Model file for the job. Use its own axes, mm. A direction names the side the tool comes from. Round coordinates to 2 decimals unless told otherwise and drop trailing zeros. Order: outer loops, then holes, each group sorted by start corner. A loop starts at its lowest first (then second) coordinate and runs counter-clockwise, first axis right, second up. Notation, with made-up numbers: (25.25, 49) -> (47.25, 49) arc R24 ccw to (47.25, 61) -> close; hole circle Ø6 at (14.5, -35). An arc over 180 degrees is marked (long way). Use CSV: the item, a comma, the result in double quotes.
```python
from build123d import *

# Parameters (mm, degrees)
SKIZZE2_W                        = 120
SKIZZE2_H                        = 39.364160046
AUFSATZ_LINEAR_AUSTRAGEN1_DEPTH  = 30
SKIZZE24_R                       = 1.55
SCHNITT_LINEAR_AUSTRAGEN4_DEPTH  = 130.805766806
SKIZZE46_R                       = 2.85
SCHNITT_LINEAR_AUSTRAGEN15_DEPTH = 10
SCHNITT_LINEAR_START             = -5
SCHNITT_LINEAR_AUSTRAGEN25_DEPTH = 2.7
LINEARES_MUSTER1_COUNT           = 4
LINEARES_MUSTER1_PITCH           = 20
SPIEGELN2_COPY_1_SKETCH_R        = 2.85
SPIEGELN2_COPY_1_DEPTH           = 10
SPIEGELN2_COPY_2_SKETCH_R        = 2.85
SPIEGELN2_COPY_2_DEPTH           = 10
SPIEGELN2_COPY_3_SKETCH_R        = 2.85
SPIEGELN2_COPY_3_DEPTH           = 10
SPIEGELN2_START                  = -5
SPIEGELN2_COPY_4_DEPTH           = 2.7
SPIEGELN2_COPY_5_DEPTH           = 2.7
SPIEGELN2_COPY_6_DEPTH           = 2.7
SKIZZE51_R                       = 1.55
SCHNITT_LINEAR_AUSTRAGEN26_DEPTH = 130.805766806
SKIZZE75_R                       = 0.75
SCHNITT_LINEAR_AUSTRAGEN28_DEPTH = 10
SKIZZE76_R                       = 2
SCHNITT_LINEAR_AUSTRAGEN29_DEPTH = 6
SKIZZE80_R                       = 0.5
SCHNITT_LINEAR_AUSTRAGEN34_DEPTH = 21
SCHNITT_LINEAR_START_2           = -7.5
SKIZZE81_R                       = 0.5
SCHNITT_LINEAR_AUSTRAGEN36_DEPTH = 5
ABSPALTEN3_OUTLINE_W             = 120
ABSPALTEN3_OUTLINE_H             = 39.364160046
ABSPALTEN3_OUTLINE_R             = 1.55
ABSPALTEN3_DEPTH                 = 15


# Read off the part's stored shape, not the designer's step: Abspalten3
with BuildPart() as part:
    # Skizze2 → Aufsatz-Linear austragen1 (new body)
    with BuildSketch(Plane.XY):
        with Locations((60, 19.682080023)):
            Rectangle(SKIZZE2_W, SKIZZE2_H)
    extrude(amount=AUFSATZ_LINEAR_AUSTRAGEN1_DEPTH)

    # Skizze24 → Schnitt-Linear austragen4 (cut, through all)
    with BuildSketch(Plane.XY.offset(30)):
        with Locations((40, 31.364160046)):
            Circle(SKIZZE24_R)
        with Locations((60, 31.364160046)):
            Circle(SKIZZE24_R)
        with Locations((80, 31.364160046)):
            Circle(SKIZZE24_R)
        with Locations((100, 31.364160046)):
            Circle(SKIZZE24_R)
    schnitt_linear_austragen4 = extrude(amount=-SCHNITT_LINEAR_AUSTRAGEN4_DEPTH, mode=Mode.SUBTRACT)

    # Skizze46 → Schnitt-Linear austragen15 (cut)
    with BuildSketch(Plane(origin=(0, 0, 0), x_dir=(-1, 0, 0), z_dir=(0, 0, -1))):
        with Locations((-100, 31.364160046)):
            Circle(SKIZZE46_R)
    schnitt_linear_austragen15 = extrude(amount=-SCHNITT_LINEAR_AUSTRAGEN15_DEPTH, mode=Mode.SUBTRACT)

    # Skizze50 → Schnitt-Linear austragen25 (cut)
    with BuildSketch(Plane.XY.offset(30).offset(SCHNITT_LINEAR_START)):
        Polygon((97.15, 33.009608314), (97.15, 39.364160046), (102.85, 39.364160046), (102.85, 33.009608314), (102.85, 29.718711779), (100, 28.073263512), (97.15, 29.718711779), align=None)
    schnitt_linear_austragen25 = extrude(amount=-SCHNITT_LINEAR_AUSTRAGEN25_DEPTH, mode=Mode.SUBTRACT)

    # Lineares Muster1: Schnitt-Linear austragen15, Schnitt-Linear austragen25 ×4
    with Locations(*[(-i * LINEARES_MUSTER1_PITCH, 0, 0) for i in range(1, LINEARES_MUSTER1_COUNT)]):
        add(schnitt_linear_austragen15, mode=Mode.SUBTRACT)
        add(schnitt_linear_austragen25, mode=Mode.SUBTRACT)

    # Spiegeln2: Schnitt-Linear austragen15, Schnitt-Linear austragen25 across plane
    add(schnitt_linear_austragen15.mirror(Plane.ZX.offset(19.764160046)), mode=Mode.SUBTRACT)
    add(schnitt_linear_austragen25.mirror(Plane.ZX.offset(19.764160046)), mode=Mode.SUBTRACT)

    # Spiegeln2 copy 1 sketch → Spiegeln2 copy 1 (cut)
    with BuildSketch(Plane(origin=(-20, 39.528320093, 0), x_dir=(-1, 0, 0), z_dir=(0, 0, -1))):
        with Locations((-100, -31.364160046)):
            Circle(SPIEGELN2_COPY_1_SKETCH_R)
    extrude(amount=-SPIEGELN2_COPY_1_DEPTH, mode=Mode.SUBTRACT)

    # Spiegeln2 copy 2 sketch → Spiegeln2 copy 2 (cut)
    with BuildSketch(Plane(origin=(-40, 39.528320093, 0), x_dir=(-1, 0, 0), z_dir=(0, 0, -1))):
        with Locations((-100, -31.364160046)):
            Circle(SPIEGELN2_COPY_2_SKETCH_R)
    extrude(amount=-SPIEGELN2_COPY_2_DEPTH, mode=Mode.SUBTRACT)

    # Spiegeln2 copy 3 sketch → Spiegeln2 copy 3 (cut)
    with BuildSketch(Plane(origin=(-60, 39.528320093, 0), x_dir=(-1, 0, 0), z_dir=(0, 0, -1))):
        with Locations((-100, -31.364160046)):
            Circle(SPIEGELN2_COPY_3_SKETCH_R)
    extrude(amount=-SPIEGELN2_COPY_3_DEPTH, mode=Mode.SUBTRACT)

    # Spiegeln2 copy 4 sketch → Spiegeln2 copy 4 (cut)
    with BuildSketch(Plane(origin=(-20, 39.528320093, 30), x_dir=(1, 0, 0), z_dir=(0, 0, 1)).offset(SPIEGELN2_START)):
        Polygon((97.15, -33.009608314), (97.15, -39.364160046), (102.85, -39.364160046), (102.85, -33.009608314), (102.85, -29.718711779), (100, -28.073263512), (97.15, -29.718711779), align=None)
    extrude(amount=-SPIEGELN2_COPY_4_DEPTH, mode=Mode.SUBTRACT)

    # Spiegeln2 copy 5 sketch → Spiegeln2 copy 5 (cut)
    with BuildSketch(Plane(origin=(-40, 39.528320093, 30), x_dir=(1, 0, 0), z_dir=(0, 0, 1)).offset(SPIEGELN2_START)):
        Polygon((97.15, -33.009608314), (97.15, -39.364160046), (102.85, -39.364160046), (102.85, -33.009608314), (102.85, -29.718711779), (100, -28.073263512), (97.15, -29.718711779), align=None)
    extrude(amount=-SPIEGELN2_COPY_5_DEPTH, mode=Mode.SUBTRACT)

    # Spiegeln2 copy 6 sketch → Spiegeln2 copy 6 (cut)
    with BuildSketch(Plane(origin=(-60, 39.528320093, 30), x_dir=(1, 0, 0), z_dir=(0, 0, 1)).offset(SPIEGELN2_START)):
        Polygon((97.15, -33.009608314), (97.15, -39.364160046), (102.85, -39.364160046), (102.85, -33.009608314), (102.85, -29.718711779), (100, -28.073263512), (97.15, -29.718711779), align=None)
    extrude(amount=-SPIEGELN2_COPY_6_DEPTH, mode=Mode.SUBTRACT)

    # Spiegeln3: Schnitt-Linear austragen4 across plane
    add(schnitt_linear_austragen4.mirror(Plane.ZX.offset(19.764160046)), mode=Mode.SUBTRACT)

    # Skizze51 → Schnitt-Linear austragen26 (cut, through all)
    with BuildSketch(Plane.XY.offset(30)):
        with Locations((5, 34.364160046)):
            Circle(SKIZZE51_R)
        with Locations((115, 5)):
            Circle(SKIZZE51_R)
    extrude(amount=-SCHNITT_LINEAR_AUSTRAGEN26_DEPTH, mode=Mode.SUBTRACT)

    # Skizze73 → Schnitt-Rotation5 (revolve, cut)
    with BuildSketch(Plane.XY.offset(15)):
        Polygon((15, 19.764160046), (15, 23.764160046), (20, 23.764160046), (20, 24.764160046), (100, 23.182080023), (100, 22.182080023), (105, 22.182080023), (105, 19.682080023), align=None)
    revolve(axis=Axis((105, 19.682080023, 15), (-0.9999995841280241, 0.0009119998787298228, 0)), mode=Mode.SUBTRACT)

    # Skizze75 → Schnitt-Linear austragen28 (cut)
    with BuildSketch(Plane.XY.offset(30)):
        with Locations((21.598259807, 19.682080023)):
            Circle(SKIZZE75_R)
    extrude(amount=-SCHNITT_LINEAR_AUSTRAGEN28_DEPTH, mode=Mode.SUBTRACT)

    # Skizze76 → Schnitt-Linear austragen29 (cut)
    with BuildSketch(Plane.XY.offset(30)):
        with Locations((21.598259807, 19.682080023)):
            Circle(SKIZZE76_R)
    extrude(amount=-SCHNITT_LINEAR_AUSTRAGEN29_DEPTH, mode=Mode.SUBTRACT)

    # Skizze80 → Schnitt-Linear austragen34 (cut)
    with BuildSketch(Plane(origin=(120, 0, 0), x_dir=(0, 0, -1), z_dir=(1, 0, 0))):
        with Locations((-22.000416524, 19.763714623)):
            Circle(SKIZZE80_R)
    schnitt_linear_austragen34 = extrude(amount=-SCHNITT_LINEAR_AUSTRAGEN34_DEPTH, mode=Mode.SUBTRACT)

    # Skizze81 → Schnitt-Linear austragen36 (cut)
    with BuildSketch(Plane.XY.offset(30).offset(SCHNITT_LINEAR_START_2)):
        with Locations(Location((99, 19.682080023, 0), (0, 0, 7.034090001))):
            Circle(SKIZZE81_R)
    schnitt_linear_austragen36 = extrude(amount=-SCHNITT_LINEAR_AUSTRAGEN36_DEPTH, mode=Mode.SUBTRACT)

    # Spiegeln4: Schnitt-Linear austragen34, Schnitt-Linear austragen36 across plane
    add(schnitt_linear_austragen34.mirror(Plane.XY.offset(15)), mode=Mode.SUBTRACT)
    add(schnitt_linear_austragen36.mirror(Plane.XY.offset(15)), mode=Mode.SUBTRACT)

    # Abspalten3 outline → Abspalten3 (cut)
    with BuildSketch(Plane.XY):
        with Locations((60, 19.682080023)):
            Rectangle(ABSPALTEN3_OUTLINE_W, ABSPALTEN3_OUTLINE_H)
        with Locations((115, 5)):
            Circle(ABSPALTEN3_OUTLINE_R, mode=Mode.SUBTRACT)
        with Locations((5, 34.364160046)):
            Circle(ABSPALTEN3_OUTLINE_R, mode=Mode.SUBTRACT)
        with Locations((40, 8.164160046)):
            Circle(ABSPALTEN3_OUTLINE_R, mode=Mode.SUBTRACT)
        with Locations((60, 8.164160046)):
            Circle(ABSPALTEN3_OUTLINE_R, mode=Mode.SUBTRACT)
        with Locations((80, 8.164160046)):
            Circle(ABSPALTEN3_OUTLINE_R, mode=Mode.SUBTRACT)
        with Locations((100, 8.164160046)):
            Circle(ABSPALTEN3_OUTLINE_R, mode=Mode.SUBTRACT)
        with Locations((40, 31.364160046)):
            Circle(ABSPALTEN3_OUTLINE_R, mode=Mode.SUBTRACT)
        with Locations((100, 31.364160046)):
            Circle(ABSPALTEN3_OUTLINE_R, mode=Mode.SUBTRACT)
        with Locations((60, 31.364160046)):
            Circle(ABSPALTEN3_OUTLINE_R, mode=Mode.SUBTRACT)
        with Locations((80, 31.364160046)):
            Circle(ABSPALTEN3_OUTLINE_R, mode=Mode.SUBTRACT)
    extrude(amount=ABSPALTEN3_DEPTH, mode=Mode.SUBTRACT)


solid = part.part
```
Q1. Pin check, flat tips, straight feed: pin 1 (2.5 mm diameter, centred on x = 100, y = 8.16, fed in from -Z); pin 2 (5 mm diameter, centred on x = 21.6, y = 19.68, fed in from -Z). Stop position of each tip, or through.
From the geometry:
pin 1,"passes through"
pin 2,"stops at z = 18.47"
Q2. Mould opens along X. For faces 4 (the flat face through (0, 19, 22)), 5 (the flat face through (59.2, 24.3, 15)), 6 (the flat face through (61.445, 10.621, 23.669)) say: +X half, -X half, draft (parallel to the pull), parting line (faces both ways), or undercut.
From the geometry:
face 4,"-X half"
face 5,"draft"
face 6,"undercut"
Q3. Cut at A-A (y = 5). Give the cut face in (x, z), plus the area to 3 significant figures.
From the geometry:
outline,"(0, 15) -> (113.45, 15) -> (113.45, 30) -> (0, 30) -> close; (116.55, 15) -> (120, 15) -> (120, 30) -> (116.55, 30) -> close; hole (37.15, 22.3) -> (42.85, 22.3) -> (42.85, 25) -> (37.15, 25) -> close; hole (57.15, 22.3) -> (62.85, 22.3) -> (62.85, 25) -> (57.15, 25) -> close; hole (77.15, 22.3) -> (82.85, 22.3) -> (82.85, 25) -> (77.15, 25) -> close; hole (97.15, 22.3) -> (102.85, 22.3) -> (102.85, 25) -> (97.15, 25) -> close"
area,"1,690 mm²"
Q4. Cut at B-B (x = 115). Give the cut face in (y, z), plus the area to 3 significant figures.
From the geometry:
outline,"(0, 15) -> (3.45, 15) -> (3.45, 30) -> (0, 30) -> close; (6.55, 15) -> (39.36, 15) -> (39.36, 30) -> (6.55, 30) -> close; hole circle Ø1 at (19.76, 22)"
area,"543 mm²"
Q5. Cut at C-C (z = 26.75). State how many separate pieces and enclosed holes the cut face has, plus the area to 3 significant figures.
From the geometry:
separate pieces,"1"
enclosed holes,"11"
area,"4,640 mm²"
Q6. Probe line 1 along Y through (x, z) = (60, 19.75); line 2 along X through (y, z) = (8, 24.25); line 3 along X through (y, z) = (34.5, 21.5). List the from-to ranges inside material, lowest first.
From the geometry:
line 1,"y = 0 to 6.61, 9.71 to 29.81, 32.91 to 39.36"
line 2,"x = 0 to 37.15, 42.85 to 57.15, 62.85 to 77.15, 82.85 to 97.15, 102.85 to 120"
line 3,"x = 0 to 3.46, 6.54 to 120"
Q7. Which spindle directions (+Z, -Z, +X, -X, +Y, -Y) get a long thin tool onto all of the face, cutting with end or side? Do faces 1 (the flat face through (100, 4, 25)), 2 (the flat face through (97.15, 35, 24)), 3 (the cylindrical face through (61.48, 7.7, 27.54)). Say none if no direction does.
From the geometry:
face 1,"none"
face 2,"+Y"
face 3,"+Z, -Z"
